from build123d import *

# Parameters (mm, degrees)
F0_W     = 42.3
F0_H     = 30
F0_R     = 10.65
F1_DEPTH = 60
F3_DEPTH = 30
F4_R     = 3.55
F5_DEPTH = 4
F7_DEPTH = 60


with BuildPart() as f1:
    # F0 (on Front) → F1 (new body)
    with BuildSketch(Plane.XZ):
        with Locations((0, -0.15)):
            Rectangle(F0_W, F0_H)
        Circle(F0_R, mode=Mode.SUBTRACT)
    extrude(amount=F1_DEPTH)

    # F2 (on face) → F3 (cut)
    with BuildSketch(Plane(origin=(0, 0, -15.15), x_dir=(1, 0, 0), z_dir=(0, 0, -1))):
        with BuildLine():
            ThreePointArc((-15.1, 52.05), (-16.549569, 48.550431), (-13.05, 50))
            ThreePointArc((-13.05, 50), (-13.650431, 51.449569), (-15.1, 52.05))
        make_face()
        with BuildLine():
            ThreePointArc((15.1, 52.05), (13.650431, 48.550431), (17.15, 50))
            ThreePointArc((17.15, 50), (16.549569, 51.449569), (15.1, 52.05))
        make_face()
        with BuildLine():
            ThreePointArc((-15.1, 7.95), (-13.650431, 8.550431), (-13.05, 10))
            ThreePointArc((-13.05, 10), (-16.549569, 11.449569), (-15.1, 7.95))
        make_face()
        with BuildLine():
            ThreePointArc((15.1, 7.95), (16.549569, 8.550431), (17.15, 10))
            ThreePointArc((17.15, 10), (13.650431, 11.449569), (15.1, 7.95))
        make_face()
    extrude(amount=-F3_DEPTH, mode=Mode.SUBTRACT)

    # F4 (on face) → F5 (cut)
    with BuildSketch(Plane(origin=(0, 0, -15.15), x_dir=(1, 0, 0), z_dir=(0, 0, -1))):
        with Locations((-15.1, 50)):
            Circle(F4_R)
        with Locations((15.1, 50)):
            Circle(F4_R)
        with Locations((-15.1, 10)):
            Circle(F4_R)
        with Locations((15.1, 10)):
            Circle(F4_R)
    extrude(amount=-F5_DEPTH, mode=Mode.SUBTRACT)

    # F6 (on face) → F7 (cut)
    with BuildSketch(Plane(origin=(0, 0, 0), x_dir=(-1, 0, 0), z_dir=(0, 1, 0))):
        with BuildLine():
            Line((21.15, -0.5), (21.15, 0))
            Line((21.15, 0), (10.65, 0))
            ThreePointArc((10.65, 0), (10.647064, -0.250069), (10.638256, -0.5))
            Line((10.638256, -0.5), (21.15, -0.5))
        make_face()
        with BuildLine():
            Line((10.65, 0), (21.15, 0))
            Line((21.15, 0), (21.15, 0.5))
            Line((21.15, 0.5), (10.638256, 0.5))
            ThreePointArc((10.638256, 0.5), (10.647064, 0.250069), (10.65, 0))
        make_face()
    extrude(amount=-F7_DEPTH, mode=Mode.SUBTRACT)


solid = f1.part
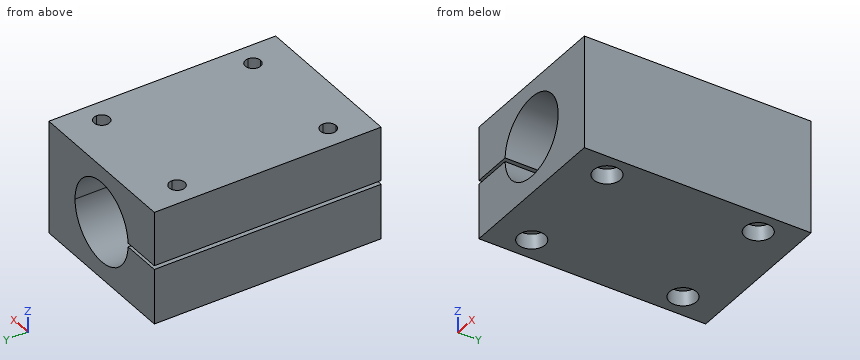
Could you check a few things on this model? Use its own coordinates, in mm. Give positions to 0.01 mm unless a question says otherwise; leave off trailing zeros. Write each loop counter-clockwise with the first axis right and the second up, starting at its lowest first coordinate (ties: lowest second). Pieces come first, ordered by that corner, then holes. Notation, with made-up numbers: (11.5, -14) -> (49.5, -14) arc R31 cw to (49.5, 19) -> close; hole circle Ø7 at (-16, 63). An arc over 180 degrees is marked (long way). Write each question's results on one line, items separated by ' | '. Start each with the question number.
Q1. Suppose I cut it at D-D, the plane z = 8. List the corners of the cut face in (x, y) for me, and give its area (3 significant figures).
Q2. I need wall thicknesses on probe 1 along Y at (x, z) = (-15.1, -12.1); probe 2 along Y at (x, z) = (-15.1, 12.25); probe 3 along X at (y, z) = (-50, -14.15). Which ranges of each line are inside material? Lowest first, please.
Q3. Suppose I cut it at A-A, the plane z = 3.25. List the corners of the cut face in (x, y) for me, and give its area (3 significant figures).
Q4. Suppose I cut it at C-C, the plane y = -33. List the corners of the cut face in (x, z) for me, and give its area (3 significant figures).
Q5. I'm going to push a flat-ended pin straight in: pin 1 Ø4.5 at (x, y) = (-15.1, -50) entering from -Z. Where does the tip first touch, or does it pass through?
Q6. Suppose I cut it at B-B, the plane x = 3. List the corners of the cut face in (y, z) for me.
Outcome:
1) outline: (-21.15, -60) -> (-7.03, -60) -> (-7.03, 0) -> (-21.15, 0) -> close; (7.03, -60) -> (21.15, -60) -> (21.15, 0) -> (7.03, 0) -> close; hole circle Ø4.1 at (-15.1, -50); hole circle Ø4.1 at (-15.1, -10); hole circle Ø4.1 at (15.1, -50); hole circle Ø4.1 at (15.1, -10) | area: 1,640 mm2
2) probe 1: -60 to -53.55, -46.45 to -13.55, -6.45 to 0 | probe 2: -60 to -52.05, -47.95 to -12.05, -7.95 to 0 | probe 3: -21.15 to -18.65, -11.55 to 11.55, 18.65 to 21.15
3) outline: (-21.15, -60) -> (-10.14, -60) -> (-10.14, 0) -> (-21.15, 0) -> close; (10.14, -60) -> (21.15, -60) -> (21.15, 0) -> (10.14, 0) -> close; hole circle Ø4.1 at (-15.1, -50); hole circle Ø4.1 at (-15.1, -10); hole circle Ø4.1 at (15.1, -50); hole circle Ø4.1 at (15.1, -10) | area: 1,270 mm2
4) outline: (-21.15, -15.15) -> (21.15, -15.15) -> (21.15, 14.85) -> (-21.15, 14.85) -> (-21.15, 0.5) -> (-10.64, 0.5) arc R10.65 cw (long way) to (-10.64, -0.5) -> (-21.15, -0.5) -> close | area: 902 mm2
5) pin 1: z = -11.15
6) outline: (-60, -15.15) -> (0, -15.15) -> (0, -10.22) -> (-60, -10.22) -> close; (-60, 10.22) -> (0, 10.22) -> (0, 14.85) -> (-60, 14.85) -> close
